Geometry: final body of the model. Coordinates: model frame, mm. A direction names the side the tool comes from. Coordinates: 2 decimals unless noted, no trailing zeros. Loops run counter-clockwise (first coordinate to the right, second up) from the corner with the lowest first, then second, coordinate; pieces in that order, holes last. Notation, with made-up numbers: (0, 19.25) - (49, 19.25) arc R18 cw to (49, 50.25) - close; hole circle Ø2 at (31, 21.25). An arc over 180 degrees is marked (long way). Return JSON: item names as keys, results as strings.
from build123d import *

# Parameters (mm, degrees)
SKETCH1_W           = 228.6
SKETCH1_H           = 63.5
BOSS_EXTRUDE1_DEPTH = 6.35
SKETCH3_R           = 7.8
SKETCH3_W           = 20
SKETCH3_H           = 6.35
SKETCH3_W_2         = 10
SKETCH3_H_2         = 2
CUT_EXTRUDE1_DEPTH  = 119.79762203
CUT_EXTRUDE2_DEPTH  = 119.79762203


with BuildPart() as part:
    # Sketch1 → Boss-Extrude1 (new body)
    with BuildSketch(Plane.XY):
        Rectangle(SKETCH1_W, SKETCH1_H)
    extrude(amount=BOSS_EXTRUDE1_DEPTH)

    # Sketch3 → Cut-Extrude1 (cut, through all)
    with BuildSketch(Plane.XY.offset(6.35)):
        with Locations((-34.3, 0)):
            Circle(SKETCH3_R)
        with Locations((-9.3, 0)):
            Circle(SKETCH3_R)
        with Locations((15.7, 0)):
            Circle(SKETCH3_R)
        with Locations((40.7, 0)):
            Circle(SKETCH3_R)
        with Locations((65.7, 0)):
            Circle(SKETCH3_R)
        with Locations((-104.3, -28.575)):
            Rectangle(SKETCH3_W, SKETCH3_H)
        with Locations((0, -28.575)):
            Rectangle(SKETCH3_W, SKETCH3_H)
        with Locations((104.3, -28.575)):
            Rectangle(SKETCH3_W, SKETCH3_H)
        with Locations((-9.3, -15)):
            Rectangle(SKETCH3_W_2, SKETCH3_H_2)
        with Locations((-34.3, -15)):
            Rectangle(SKETCH3_W_2, SKETCH3_H_2)
        with Locations((15.7, -15)):
            Rectangle(SKETCH3_W_2, SKETCH3_H_2)
        with Locations((40.7, -15)):
            Rectangle(SKETCH3_W_2, SKETCH3_H_2)
        with Locations((65.7, -15)):
            Rectangle(SKETCH3_W_2, SKETCH3_H_2)
    extrude(amount=-CUT_EXTRUDE1_DEPTH, mode=Mode.SUBTRACT)

    # Sketch5 → Cut-Extrude2 (cut, through all)
    with BuildSketch(Plane(origin=(0, 0, 0), x_dir=(-1, 0, 0), z_dir=(0, 0, -1))):
        Polygon((93.861415546, -7.039545532), (66.361415546, -7.039545532), (66.361415546, 7.169080451), (71.505824709, 12.260454468), (88.717006383, 12.260454468), (93.861415546, 7.169080451), align=None)
    extrude(amount=-CUT_EXTRUDE2_DEPTH, mode=Mode.SUBTRACT)


solid = part.part
Item 1: Reachability of faces 4 (the face through (10, -29, 3)), 5 (the face through (-9, -16, 3)), 6 (the face through (104, -25.4, 3)), 7 (the face through (-2, 8, 0)) from +Z, -Z, +X, -X, +Y, -Y: full face, straight path, thin tool, end or side. Return the list, or none.
Worked out:
{"face 4": "+Z, -Z, -Y", "face 5": "+Z, -Z", "face 6": "+Z, -Z, +X, -Y", "face 7": "-Z, +X, -X, +Y, -Y"}
Item 2: First-contact query: pin 1 Ø20.5 at (x, y) = (40.7, 0) entering from -Z; pin 2 Ø3 at (x, z) = (-103, 4) entering from -Y; pin 3 Ø3 at (y, z) = (-28.5, 2.5) entering from +X; pin 4 Ø9.5 at (x, y) = (-34.3, 0) entering from +Z. Flat tips, straight axial feed; report the tip coordinate or a pass-through.
Worked out:
{"pin 1": "z = 0", "pin 2": "y = -25.4", "pin 3": "x = 94.3", "pin 4": "through"}
Item 3: Section query B-B, the plane x = -83.5. Return loops of the section in (y, z), and give its area (3 significant figures).
Worked out:
{"outline": "(-31.75, 0) - (-7.04, 0) - (-7.04, 6.35) - (-31.75, 6.35) - close; (12.26, 0) - (31.75, 0) - (31.75, 6.35) - (12.26, 6.35) - close", "area": "281 mm^2"}
Item 4: Section query C-C, the plane x = 40.7. Return loops of the section in (y, z), and give its area (3 significant figures).
Worked out:
{"outline": "(-31.75, 0) - (-16, 0) - (-16, 6.35) - (-31.75, 6.35) - close; (-14, 0) - (-7.8, 0) - (-7.8, 6.35) - (-14, 6.35) - close; (7.8, 0) - (31.75, 0) - (31.75, 6.35) - (7.8, 6.35) - close", "area": "291 mm^2"}
Item 5: Section query D-D, the plane z = 1.25. Count the separate pieces of the cut face and the enclosed holes in it, and give its area (3 significant figures).
Worked out:
{"separate pieces": "1", "enclosed holes": "11", "area": "12,600 mm^2"}
Item 6: Ray query, probe 1 along Y at (x, z) = (15.7, 4.25); probe 2 along Y at (x, z) = (-72, 5.5); probe 3 along Y at (x, z) = (43, 5). Return the intervals inside material, ascending. Write a range as from..to.
Worked out:
{"probe 1": "-31.75..-16, -14..-7.8, 7.8..31.75", "probe 2": "-31.75..-7.04, 12.26..31.75", "probe 3": "-31.75..-16, -14..-7.45, 7.45..31.75"}
Item 7: Section query A-A, the plane y = 0. Return loops of the section in (x, z), and give its area (3 significant figures).
Worked out:
{"outline": "(-114.3, 0) - (-93.86, 0) - (-93.86, 6.35) - (-114.3, 6.35) - close; (-66.36, 0) - (-42.1, 0) - (-42.1, 6.35) - (-66.36, 6.35) - close; (-26.5, 0) - (-17.1, 0) - (-17.1, 6.35) - (-26.5, 6.35) - close; (-1.5, 0) - (7.9, 0) - (7.9, 6.35) - (-1.5, 6.35) - close; (23.5, 0) - (32.9, 0) - (32.9, 6.35) - (23.5, 6.35) - close; (48.5, 0) - (57.9, 0) - (57.9, 6.35) - (48.5, 6.35) - close; (73.5, 0) - (114.3, 0) - (114.3, 6.35) - (73.5, 6.35) - close", "area": "782 mm^2"}
Item 8: Mould query, pull axis X, two halves, no side actions, for faces 1 (the face through (-34, -16, 3)), 2 (the face through (94.3, -29, 3)), 3 (the face through (-2, 8, 6.35)). Classes: +X half, -X half, draft (parallel to the pull), parting line (faces both ways), or undercut.
Worked out:
{"face 1": "undercut", "face 2": "+X half", "face 3": "draft"}
